from build123d import *

# Parameters (mm, degrees)
BOSS_EXTRUDE1_DEPTH     = 3
BOSS_EXTRUDE2_DEPTH     = 64.08
BOSS_EXTRUDE3_START     = 0.3
BOSS_EXTRUDE3_DEPTH     = 3
CUT_EXTRUDE1_REACH      = 5
SKETCH4_R               = 1.65
CUT_EXTRUDE2_DEPTH      = 2
CUT_EXTRUDE3_REACH      = 5
SKETCH7_R               = 1.6
SKETCH10_W              = 10
SKETCH10_H              = 10
CUT_EXTRUDE4_DEPTH      = 38
CUT_EXTRUDE4_DEPTH_BACK = 4
CUT_EXTRUDE6_DEPTH      = 1.5
CUT_EXTRUDE7_REACH      = 5
SKETCH12_R              = 1.6
CUT_EXTRUDE8_REACH      = 87.591
BOSS_EXTRUDE4_DEPTH     = 3.3
CUT_EXTRUDE9_REACH      = 5.3
SKETCH15_R              = 1.6
CUT_EXTRUDE10_DEPTH     = 1.5
SKETCH17_R              = 8
CUT_EXTRUDE11_DEPTH     = 1
SKETCH18_R              = 2.75
CUT_EXTRUDE13_DEPTH     = 1
FILLET1_R               = 2
FILLET2_R               = 5


with BuildPart() as part:
    # Sketch1 → Boss-Extrude1 (new body)
    with BuildSketch(Plane.XY):
        with BuildLine():
            Line((-85.590530374, -20.367507575), (-53.15, -20.367507575))
            ThreePointArc((-53.15, -20.367507575), (-33.15, -0.367507575), (-53.15, 19.632492425))
            Line((-53.15, 19.632492425), (-85.590530374, 19.632492425))
            Line((-85.590530374, 19.632492425), (-85.590530374, -20.367507575))
        make_face()
    extrude(amount=BOSS_EXTRUDE1_DEPTH)

    # Sketch2 → Boss-Extrude2 (add)
    with BuildSketch(Plane.XY.offset(3)):
        with BuildLine():
            Line((-85.590530374, -20.367507575), (-53.15, -20.367507575))
            ThreePointArc((-53.15, -20.367507575), (-33.15, -0.367507575), (-53.15, 19.632492425))
            Line((-53.15, 19.632492425), (-85.590530374, 19.632492425))
            Line((-85.590530374, 19.632492425), (-85.590530374, 16.632492425))
            Line((-85.590530374, 16.632492425), (-53.15, 16.632492425))
            ThreePointArc((-53.15, 16.632492425), (-36.15, -0.367507575), (-53.15, -17.367507575))
            Line((-53.15, -17.367507575), (-85.590530374, -17.367507575))
            Line((-85.590530374, -17.367507575), (-85.590530374, -20.367507575))
        make_face()
    extrude(amount=BOSS_EXTRUDE2_DEPTH)

    # Sketch3 → Boss-Extrude3 (add)
    with BuildSketch(Plane(origin=(0, 0, 67.38), x_dir=(-1, 0, 0), z_dir=(0, 0, -1)).offset(BOSS_EXTRUDE3_START)):
        with BuildLine():
            Line((85.590530374, 19.632492425), (85.590530374, 11.632492425))
            Line((85.590530374, 11.632492425), (77.590530374, 11.632492425))
            Line((77.590530374, 11.632492425), (53.15, 11.632492425))
            ThreePointArc((53.15, 11.632492425), (41.15, -0.367507575), (53.15, -12.367507575))
            Line((53.15, -12.367507575), (77.590530374, -12.367507575))
            Line((77.590530374, -12.367507575), (85.590530374, -12.367507575))
            Line((85.590530374, -12.367507575), (85.590530374, -20.367507575))
            Line((85.590530374, -20.367507575), (53.15, -20.367507575))
            ThreePointArc((53.15, -20.367507575), (33.15, -0.367507575), (53.15, 19.632492425))
            Line((53.15, 19.632492425), (85.590530374, 19.632492425))
        make_face()
    extrude(amount=BOSS_EXTRUDE3_DEPTH)

    # Sketch4 → Cut-Extrude1 (cut, up to next)
    with BuildSketch(Plane.XY.offset(3), mode=Mode.PRIVATE) as cut_extrude1_sk1:
        with Locations((-77.35, -0.367507575)):
            Circle(SKETCH4_R)
    cut_extrude1_tool1 = extrude(cut_extrude1_sk1.sketch, amount=-CUT_EXTRUDE1_REACH, mode=Mode.PRIVATE) & part.part
    add(cut_extrude1_tool1.solids().sort_by_distance((-77.35, -0.367508, 3))[0], mode=Mode.SUBTRACT)
    # Sketch4 → Cut-Extrude1 (cut, up to next)
    with BuildSketch(Plane.XY.offset(3), mode=Mode.PRIVATE) as cut_extrude1_sk2:
        with Locations((-53.15, -0.367507575)):
            Circle(SKETCH4_R)
    cut_extrude1_tool2 = extrude(cut_extrude1_sk2.sketch, amount=-CUT_EXTRUDE1_REACH, mode=Mode.PRIVATE) & part.part
    add(cut_extrude1_tool2.solids().sort_by_distance((-53.15, -0.367508, 3))[0], mode=Mode.SUBTRACT)

    # Sketch6 → Cut-Extrude2 (cut)
    with BuildSketch(Plane.XY.offset(3)):
        Polygon((-77.715530374, -9.047743527), (-80.590530374, -10.707625551), (-80.590530374, -14.027389599), (-77.715530374, -15.687271623), (-74.840530374, -14.027389599), (-74.840530374, -10.707625551), align=None)
        Polygon((-56.965530374, -9.047743527), (-59.840530374, -10.707625551), (-59.840530374, -14.027389599), (-56.965530374, -15.687271623), (-54.090530374, -14.027389599), (-54.090530374, -10.707625551), align=None)
        Polygon((-77.715530374, 14.952256473), (-80.590530374, 13.292374449), (-80.590530374, 9.972610401), (-77.715530374, 8.312728377), (-74.840530374, 9.972610401), (-74.840530374, 13.292374449), align=None)
        Polygon((-56.965530374, 14.952256473), (-59.840530374, 13.292374449), (-59.840530374, 9.972610401), (-56.965530374, 8.312728377), (-54.090530374, 9.972610401), (-54.090530374, 13.292374449), align=None)
    extrude(amount=-CUT_EXTRUDE2_DEPTH, mode=Mode.SUBTRACT)

    # Sketch7 → Cut-Extrude3 (cut, up to next)
    with BuildSketch(Plane.XY.offset(3), mode=Mode.PRIVATE) as cut_extrude3_sk1:
        with Locations((-77.715530374, -12.367507575)):
            Circle(SKETCH7_R)
    cut_extrude3_tool1 = extrude(cut_extrude3_sk1.sketch, amount=-CUT_EXTRUDE3_REACH, mode=Mode.PRIVATE) & part.part
    add(cut_extrude3_tool1.solids().sort_by_distance((-77.71553, -12.367508, 3))[0], mode=Mode.SUBTRACT)
    # Sketch7 → Cut-Extrude3 (cut, up to next)
    with BuildSketch(Plane.XY.offset(3), mode=Mode.PRIVATE) as cut_extrude3_sk2:
        with Locations((-77.715530374, 11.632492425)):
            Circle(SKETCH7_R)
    cut_extrude3_tool2 = extrude(cut_extrude3_sk2.sketch, amount=-CUT_EXTRUDE3_REACH, mode=Mode.PRIVATE) & part.part
    add(cut_extrude3_tool2.solids().sort_by_distance((-77.71553, 11.632492, 3))[0], mode=Mode.SUBTRACT)
    # Sketch7 → Cut-Extrude3 (cut, up to next)
    with BuildSketch(Plane.XY.offset(3), mode=Mode.PRIVATE) as cut_extrude3_sk3:
        with Locations((-56.965530374, 11.632492425)):
            Circle(SKETCH7_R)
    cut_extrude3_tool3 = extrude(cut_extrude3_sk3.sketch, amount=-CUT_EXTRUDE3_REACH, mode=Mode.PRIVATE) & part.part
    add(cut_extrude3_tool3.solids().sort_by_distance((-56.96553, 11.632492, 3))[0], mode=Mode.SUBTRACT)
    # Sketch7 → Cut-Extrude3 (cut, up to next)
    with BuildSketch(Plane.XY.offset(3), mode=Mode.PRIVATE) as cut_extrude3_sk4:
        with Locations((-56.965530374, -12.367507575)):
            Circle(SKETCH7_R)
    cut_extrude3_tool4 = extrude(cut_extrude3_sk4.sketch, amount=-CUT_EXTRUDE3_REACH, mode=Mode.PRIVATE) & part.part
    add(cut_extrude3_tool4.solids().sort_by_distance((-56.96553, -12.367508, 3))[0], mode=Mode.SUBTRACT)

    # Sketch10 → Cut-Extrude4 (cut, two sides)
    with BuildSketch(Plane(origin=(0, -17.367507575, 0), x_dir=(1, 0, 0), z_dir=(0, 1, 0))) as cut_extrude4_sk:
        with Locations((-80.590530374, -59.08)):
            Rectangle(SKETCH10_W, SKETCH10_H)
    extrude(amount=CUT_EXTRUDE4_DEPTH, mode=Mode.SUBTRACT)
    extrude(cut_extrude4_sk.sketch, amount=-CUT_EXTRUDE4_DEPTH_BACK, mode=Mode.SUBTRACT)

    # Sketch11 → Cut-Extrude6 (cut)
    with BuildSketch(Plane(origin=(0, 0, 64.08), x_dir=(-1, 0, 0), z_dir=(0, 0, -1))):
        Polygon((80.590530374, 12.312728377), (83.465530374, 13.972610401), (83.465530374, 17.292374449), (80.590530374, 18.952256473), (77.715530374, 17.292374449), (77.715530374, 13.972610401), align=None)
        Polygon((80.595461682, -19.68726796), (83.467992856, -18.02311713), (83.463061548, -14.703356745), (80.585599066, -13.04774719), (77.713067892, -14.71189802), (77.7179992, -18.031658405), align=None)
    extrude(amount=-CUT_EXTRUDE6_DEPTH, mode=Mode.SUBTRACT)

    # Sketch12 → Cut-Extrude7 (cut, up to next)
    with BuildSketch(Plane(origin=(0, 0, 64.08), x_dir=(-1, 0, 0), z_dir=(0, 0, -1)), mode=Mode.PRIVATE) as cut_extrude7_sk1:
        with Locations((80.590530374, 15.632492425)):
            Circle(SKETCH12_R)
    cut_extrude7_tool1 = extrude(cut_extrude7_sk1.sketch, amount=-CUT_EXTRUDE7_REACH, mode=Mode.PRIVATE) & part.part
    add(cut_extrude7_tool1.solids().sort_by_distance((-80.59053, 15.632492, 64.08))[0], mode=Mode.SUBTRACT)
    # Sketch12 → Cut-Extrude7 (cut, up to next)
    with BuildSketch(Plane(origin=(0, 0, 64.08), x_dir=(-1, 0, 0), z_dir=(0, 0, -1)), mode=Mode.PRIVATE) as cut_extrude7_sk2:
        with Locations((80.590530374, -16.363236937)):
            Circle(SKETCH12_R)
    cut_extrude7_tool2 = extrude(cut_extrude7_sk2.sketch, amount=-CUT_EXTRUDE7_REACH, mode=Mode.PRIVATE) & part.part
    add(cut_extrude7_tool2.solids().sort_by_distance((-80.59053, -16.363237, 64.08))[0], mode=Mode.SUBTRACT)

    # Sketch13 → Cut-Extrude8 (cut, up to next)
    with BuildSketch(Plane(origin=(0, 0, 0), x_dir=(0, 0, -1), z_dir=(1, 0, 0)), mode=Mode.PRIVATE) as cut_extrude8_sk1:
        Polygon((-60.382396062, 0), (-60.382396062, -12.5), (-10.382396062, -12.5), (-10.382396062, 12.5), (-60.382396062, 12.5), align=None)
    cut_extrude8_tool1 = extrude(cut_extrude8_sk1.sketch, amount=-CUT_EXTRUDE8_REACH, mode=Mode.PRIVATE) & part.part
    add(cut_extrude8_tool1.solids().sort_by_distance((0, 0, 35.382396))[0], mode=Mode.SUBTRACT)

    # Sketch14 → Boss-Extrude4 (add)
    with BuildSketch(Plane(origin=(0, 0, 67.38), x_dir=(-1, 0, 0), z_dir=(0, 0, -1))):
        with BuildLine():
            Line((46.470700294, 3.632492425), (41.836291501, 3.632492425))
            ThreePointArc((41.836291501, 3.632492425), (41.149999808, -0.367507575), (41.836291501, -4.367507575))
            Line((41.836291501, -4.367507575), (46.470700294, -4.367507575))
            ThreePointArc((46.470700294, -4.367507575), (50.470700294, -0.367507575), (46.470700294, 3.632492425))
        make_face()
    extrude(amount=BOSS_EXTRUDE4_DEPTH)

    # Sketch15 → Cut-Extrude9 (cut, up to next)
    with BuildSketch(Plane(origin=(0, 0, 64.08), x_dir=(-1, 0, 0), z_dir=(0, 0, -1)), mode=Mode.PRIVATE) as cut_extrude9_sk1:
        with Locations((46.470700294, -0.367507575)):
            Circle(SKETCH15_R)
    cut_extrude9_tool1 = extrude(cut_extrude9_sk1.sketch, amount=-CUT_EXTRUDE9_REACH, mode=Mode.PRIVATE) & part.part
    add(cut_extrude9_tool1.solids().sort_by_distance((-46.4707, -0.367508, 64.08))[0], mode=Mode.SUBTRACT)

    # Sketch16 → Cut-Extrude10 (cut)
    with BuildSketch(Plane(origin=(0, 0, 64.08), x_dir=(-1, 0, 0), z_dir=(0, 0, -1))):
        Polygon((46.601103516, -3.684709458), (49.408683005, -1.913176014), (49.278279783, 1.40402587), (46.340297072, 2.949694308), (43.532717583, 1.178160864), (43.663120805, -2.139041019), align=None)
    extrude(amount=-CUT_EXTRUDE10_DEPTH, mode=Mode.SUBTRACT)

    # Sketch17 → Cut-Extrude11 (cut)
    with BuildSketch(Plane.XY.offset(3)):
        with Locations((-349.65, -0.367507575)):
            Circle(SKETCH17_R)
    extrude(amount=-CUT_EXTRUDE11_DEPTH, mode=Mode.SUBTRACT)

    # Sketch18 → Cut-Extrude13 (cut)
    with BuildSketch(Plane.XY.offset(3)):
        with Locations((-53.15, -0.367507575)):
            Circle(SKETCH18_R)
        with Locations((-77.35, -0.367507575)):
            Circle(SKETCH18_R)
    extrude(amount=-CUT_EXTRUDE13_DEPTH, mode=Mode.SUBTRACT)

    # Fillet1
    fillet1_edges = [part.edges().sort_by_distance(p)[0] for p in [
        (-85.590530374, 18.132492425, 54.08),
        (-85.590530374, -18.867507575, 54.08),
        (-75.590530374, 18.132492425, 54.08),
        (-75.590530374, -18.867507575, 54.08),
        (-75.590530374, 18.132492425, 64.08),
        (-75.590530374, -18.867507575, 64.08),
        (-85.590530374, 15.632492425, 64.08),
        (-85.590530374, -16.367507575, 64.08),
    ]]
    fillet(fillet1_edges, radius=FILLET1_R)

    # Fillet2
    fillet2_edges = [part.edges().sort_by_distance(p)[0] for p in [
        (-39.939600546, 12.5, 60.382396062),
        (-39.939600546, 12.5, 10.382396062),
        (-39.246070498, -12.5, 10.382396062),
        (-39.246070498, -12.5, 60.382396062),
    ]]
    fillet(fillet2_edges, radius=FILLET2_R)


solid = part.part
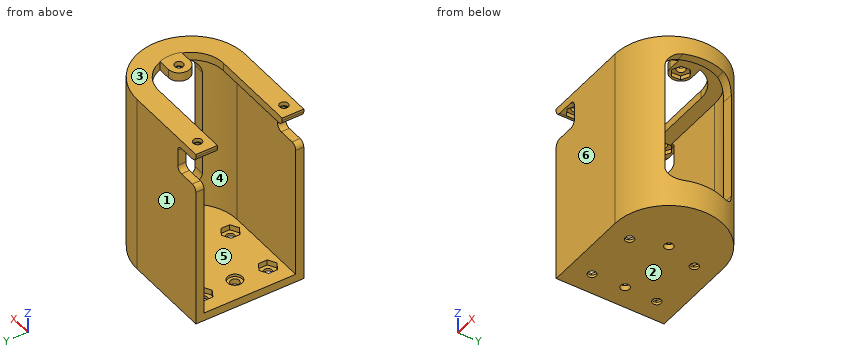
The model under review builds one solid part; all positions refer to its coordinate system, in mm. Face numbers are marked on the shaded views. A direction names the side the tool comes from. Round coordinates to 2 decimals unless told otherwise and drop trailing zeros. Loops run counter-clockwise (first coordinate to the right, second up) from the corner with the lowest first, then second, coordinate; pieces in that order, holes last. Notation, with made-up numbers: (62.5, 55) -> (106.5, 55) arc R16 ccw to (106.5, 65) -> close; hole circle Ø9 at (71, 37.25). An arc over 180 degrees is marked (long way). Write item = value, one per line. Start each with the question number.
Item 1: For the marked faces 5 and 6, list the 3-axis set-ups (+Z, -Z, +X, -X, +Y, -Y) from which the entire face can be reached by the end or side of a thin tool; tool diameter is ignored.
Item 2: Insertion check: pin 1 (6 mm diameter, centred on x = -39, z = 42.5, fed in from -Y); pin 2 (5 mm diameter, centred on y = -10.5, z = 26, fed in from +X); pin 3 (3 mm diameter, centred on x = -57.5, y = 12.5, fed in from +Z). Each pin has a flat end and moves straight along its axis. Give the tip position at first contact, or say it passes through.
Item 3: To check wall thickness, follow L1, parallel to Z at x = -51, y = 14.5; L2, parallel to Y at x = -53, z = 22; L3, parallel to Z at x = -83, y = -4. State the ranges of each line that lie inside material, in increasing order.
Item 4: Take a section at A-A on z = 32.5. Give the boundary of the cut face in (x, y).
Item 5: Mouldability with a two-part tool opening along Z and no side actions: class the marked faces 1, 2, 3 and 4 as released by +Z, released by -Z, zero draft, split by the parting line, or undercut.
Result:
q1.face_5 = -X
q1.face_6 = +Z, -Z, +X, -X, -Y
q2.pin_1 = -16.97
q2.pin_2 = -37.25
q2.pin_3 = 67.08
q3.L1 = 0 to 3, 64.08 to 67.08
q3.L2 = -20.37 to -17.37, 16.63 to 19.63
q3.L3 = 0 to 3
q4.outline = (-85.59, -20.37) -> (-53.15, -20.37) arc R20 ccw to (-37.25, -12.5) -> (-41.24, -12.5) arc R17 cw to (-53.15, -17.37) -> (-85.59, -17.37) -> close; (-85.59, 16.63) -> (-53.15, 16.63) arc R17 cw to (-42.04, 12.5) -> (-37.84, 12.5) arc R20 ccw to (-53.15, 19.63) -> (-85.59, 19.63) -> close
q5.face_1 = zero draft
q5.face_2 = released by -Z
q5.face_3 = released by +Z
q5.face_4 = undercut
